from build123d import *

# Parameters (mm, degrees)
ESQUISSE2_W             = 90
ESQUISSE2_H             = 30
BOSS_EXTRU_1_DEPTH      = 15
CONG_1_R                = 3
ESQUISSE4_W             = 20
ESQUISSE4_H             = 20
ENL_V_MAT_EXTRU_1_DEPTH = 31
ESQUISSE5_R             = 2.5
ENL_V_MAT_EXTRU_2_DEPTH = 31


with BuildPart() as part:
    # Esquisse2 → Boss.-Extru.1 (new body, symmetric)
    with BuildSketch(Plane(origin=(0, 0, 0), x_dir=(1, 0, 0), z_dir=(0, 1, 0))):
        with Locations((45, 0)):
            Rectangle(ESQUISSE2_W, ESQUISSE2_H)
    extrude(amount=BOSS_EXTRU_1_DEPTH, both=True)

    # Congé1
    cong_1_edges = [part.edges().sort_by_distance(p)[0] for p in [
        (90, 15, 0),
        (0, 15, 0),
        (90, -15, 0),
        (0, -15, 0),
    ]]
    fillet(cong_1_edges, radius=CONG_1_R)

    # Esquisse4 → Enlèv. mat.-Extru.1 (cut, through all)
    with BuildSketch(Plane(origin=(0, 15, 0), x_dir=(1, 0, 0), z_dir=(0, 1, 0))):
        with Locations((80, 0)):
            Rectangle(ESQUISSE4_W, ESQUISSE4_H)
    extrude(amount=-ENL_V_MAT_EXTRU_1_DEPTH, mode=Mode.SUBTRACT)

    # Esquisse5 → Enlèv. mat.-Extru.2 (cut, through all)
    with BuildSketch(Plane(origin=(0, 0, -15), x_dir=(-1, 0, 0), z_dir=(0, 0, -1))):
        with Locations((-85, 10)):
            Circle(ESQUISSE5_R)
        with Locations((-5, 10)):
            Circle(ESQUISSE5_R)
    extrude(amount=-ENL_V_MAT_EXTRU_2_DEPTH, mode=Mode.SUBTRACT)


solid = part.part
Here's how the part is built. I have some questions about the finished solid (model axes, mm). A direction names the side the tool comes from. Coordinates: 2 decimals unless noted, no trailing zeros. Order: outer loops, then holes, each group sorted by start corner. A loop starts at its lowest first (then second) coordinate and runs counter-clockwise, first axis right, second up. Notation, with made-up numbers: (-11.5, 48) - (29.5, 48) arc R12 ccw to (29.5, 66) - close; hole circle Ø1 at (-34, 24). An arc over 180 degrees is marked (long way). Use CSV: the item, a comma, the result in double quotes. Start each with the question number.
1. Suppose I cut it at C-C on z = -12.5. List the corners of the cut face in (x, y) for me, then the cut area to 3 significant figures.
2. Suppose I cut it at A-A on y = 10. List the corners of the cut face in (x, z) for me, then the cut area to 3 significant figures.
3. Suppose I cut it at D-D on x = 85. List the corners of the cut face in (y, z) for me.
4. If we mould it in two halves opening along X, with no side actions, what happens to faces 1 (the face through (80, 0, -10)), 2 (the face through (89.1, 14.14, 12.46)), 3 (the face through (87, 8.5, -12.5))? For each: +X half, -X half, draft (parallel to the pull), parting line (faces both ways), or undercut.
5. Suppose I cut it at B-B on x = 5. List the corners of the cut face in (y, z) for me, then the cut area to 3 significant figures.
6. For faces 4 (the face through (90, 0, 13)), 5 (the face through (70, 0, 0)), which set-ups out of +Z, -Z, +X, -X, +Y, -Y let a thin tool reach every point of the face, with its end or its side?
7. Please list where these lines run through material, in increasing order: line 1 (Z direction, x = 74, y = -7.25); line 2 (Y direction, x = 85, z = -13.55); line 3 (X direction, y = -8, z = 2.5). Write a range as from..to.
Output:
1,outline,"(0, -12) arc R3 ccw to (3, -15) - (87, -15) arc R3 ccw to (90, -12) - (90, 12) arc R3 ccw to (87, 15) - (3, 15) arc R3 ccw to (0, 12) - close; hole circle Ø5 at (5, 10); hole circle Ø5 at (85, 10)"
1,area,"2,650 mm2"
2,outline,"(0, -15) - (2.5, -15) - (2.5, 15) - (0, 15) - close; (7.5, -15) - (82.5, -15) - (82.5, -10) - (70, -10) - (70, 10) - (82.5, 10) - (82.5, 15) - (7.5, 15) - close; (87.5, -15) - (90, -15) - (90, -10) - (87.5, -10) - close; (87.5, 10) - (90, 10) - (90, 15) - (87.5, 15) - close"
2,area,"2,100 mm2"
3,outline,"(-15, -15) - (7.5, -15) - (7.5, -10) - (-15, -10) - close; (-15, 10) - (7.5, 10) - (7.5, 15) - (-15, 15) - close; (12.5, -15) - (15, -15) - (15, -10) - (12.5, -10) - close; (12.5, 10) - (15, 10) - (15, 15) - (12.5, 15) - close"
4,face 1,"draft"
4,face 2,"+X half"
4,face 3,"undercut"
5,outline,"(-15, -15) - (7.5, -15) - (7.5, 15) - (-15, 15) - close; (12.5, -15) - (15, -15) - (15, 15) - (12.5, 15) - close"
5,area,"750 mm2"
6,face 4,"+Z, -Z, +X, +Y, -Y"
6,face 5,"+X, +Y, -Y"
7,line 1,"z = -15..-10, 10..15"
7,line 2,"y = -15..7.5, 12.5..15"
7,line 3,"x = 0..70"
